The model under review builds one solid part; all positions refer to its coordinate system, in mm. Coordinates: 2 decimals unless noted, no trailing zeros. Order: outer loops, then holes, each group sorted by start corner. A loop starts at its lowest first (then second) coordinate and runs counter-clockwise, first axis right, second up. Notation, with made-up numbers: (85, 21) -> (143, 21) arc R35 ccw to (143, 60) -> close; hole circle Ø3 at (40, -5.75). An arc over 180 degrees is marked (long way). Use one line per item in the form item = value.
from build123d import *

# Parameters (mm, degrees)
SKETCH3_W           = 20
SKETCH3_H           = 10
BOSS_EXTRUDE1_DEPTH = 152.4
SKETCH4_R           = 3.125
CUT_EXTRUDE1_DEPTH  = 5


with BuildPart() as part:
    # Sketch3 → Boss-Extrude1 (new, symmetric)
    with BuildSketch(Plane.XY):
        Rectangle(SKETCH3_W, SKETCH3_H)
    extrude(amount=BOSS_EXTRUDE1_DEPTH, both=True)

    # Sketch4 → Cut-Extrude1 (cut, symmetric)
    with BuildSketch(Plane(origin=(0, 0, 0), x_dir=(1, 0, 0), z_dir=(0, 1, 0))):
        with Locations(Location((0, -44, 0), (0, 0, 270))):
            Circle(SKETCH4_R)
        with Locations(Location((0, 44, 0), (0, 0, 90))):
            Circle(SKETCH4_R)
    extrude(amount=CUT_EXTRUDE1_DEPTH, both=True, mode=Mode.SUBTRACT)


solid = part.part
Item 1: Draft analysis for pull direction X (two halves, no side actions). For faces 1 (the face through (1.197, 0.07, -46.887)), 2 (the face through (0, 0, -152.4)), 3 (the face through (10, 0, 2)), 4 (the face through (-10, 0, 2)), state which applies: released by +X, released by -X, zero draft, split by the parting line, or undercut.
Results found:
face_1 = undercut
face_2 = zero draft
face_3 = released by +X
face_4 = released by -X
Item 2: To check wall thickness, follow L1, parallel to X at y = -1.25, z = 44 (3 decimals); L2, parallel to Z at x = -0.75, y = -3.75; L3, parallel to Z at x = 1.25, y = 2. State the ranges of each line that lie inside material, in increasing order. Write a range as from..to.
Results found:
L1 = -10..-3.125, 3.125..10
L2 = -152.4..-47.03, -40.97..40.97, 47.03..152.4
L3 = -152.4..-46.86, -41.14..41.14, 46.86..152.4
Item 3: We need section A-A (x = 0). Write out the cut boundary in (y, z) (3 decimals), plus the area to 3 significant figures.
Results found:
outline = (-5, -152.4) -> (5, -152.4) -> (5, -47.125) -> (-5, -47.125) -> close; (-5, -40.875) -> (5, -40.875) -> (5, 40.875) -> (-5, 40.875) -> close; (-5, 47.125) -> (5, 47.125) -> (5, 152.4) -> (-5, 152.4) -> close
area = 2,920 mm²
Item 4: Clearance check with a flat-ended pin moving along its axis: pin 1 (4 mm diameter, centred on x = 0, z = 44, fed in from +Y). State where the tip first meets the part, or that it passes through.
Results found:
pin_1 = through
Item 5: We need section B-B (z = 44). Write out the cut boundary in (x, y) (3 decimals).
Results found:
outline = (-10, -5) -> (-3.125, -5) -> (-3.125, 5) -> (-10, 5) -> close; (3.125, -5) -> (10, -5) -> (10, 5) -> (3.125, 5) -> close
